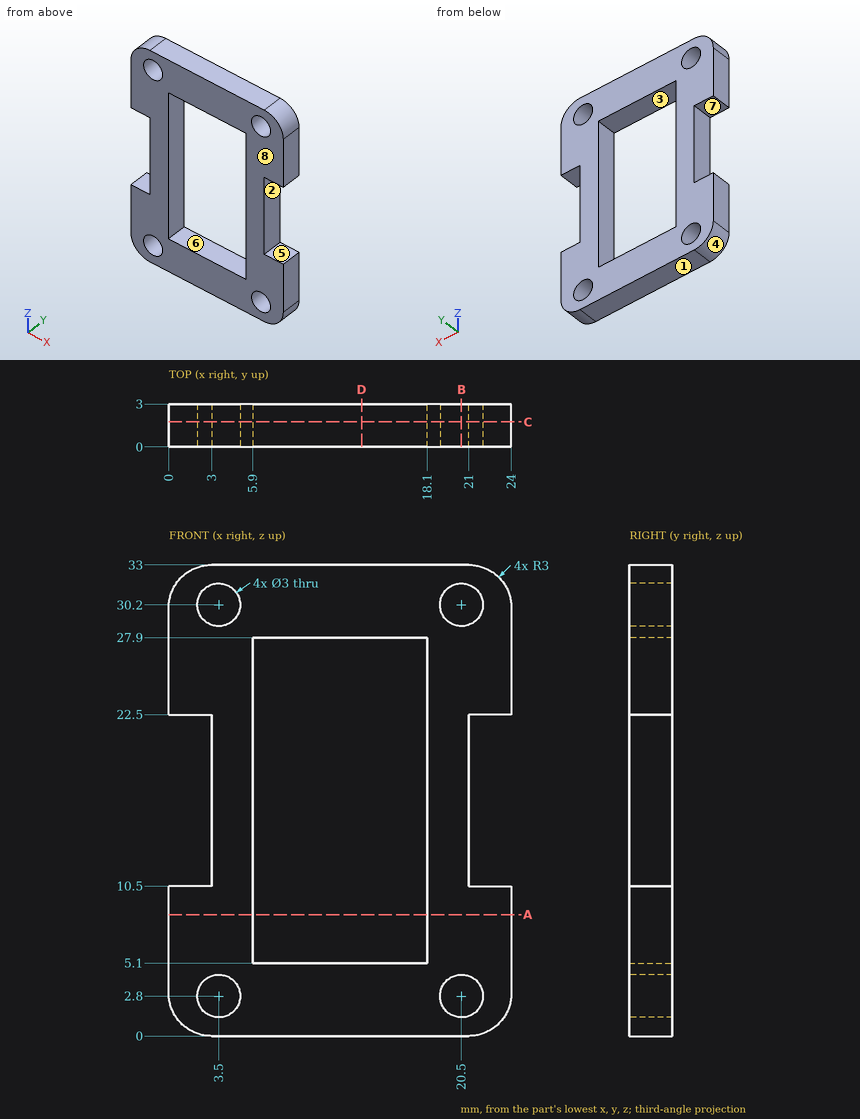
Could you check a few things on this drawing? It's one solid part, dimensions in mm from its lowest x, y, z. A direction names the side the tool comes from. Round coordinates to 2 decimals unless told otherwise and drop trailing zeros. Order: outer loops, then holes, each group sorted by start corner. A loop starts at its lowest first (then second) coordinate and runs counter-clockwise, first axis right, second up.
(1) Imagine slicing it at A-A (z = 8.5). Write out the boundary of the cut face in (x, y), plus the area to 3 significant figures.
Response values:
outline: (0, 0) - (5.9, 0) - (5.9, 3) - (0, 3) - close; (18.1, 0) - (24, 0) - (24, 3) - (18.1, 3) - close
area: 35.4 mm2
(2) Imagine slicing it at C-C (y = 1.75). Write out the boundary of the cut face in (x, z), plus the area to 3 significant figures.
Response values:
outline: (0, 3) arc R3 ccw to (3, 0) - (21, 0) arc R3 ccw to (24, 3) - (24, 10.5) - (21, 10.5) - (21, 22.5) - (24, 22.5) - (24, 30) arc R3 ccw to (21, 33) - (3, 33) arc R3 ccw to (0, 30) - (0, 22.5) - (3, 22.5) - (3, 10.5) - (0, 10.5) - close; hole circle Ø3 at (3.5, 2.8); hole circle Ø3 at (3.5, 30.2); hole (5.9, 5.1) - (18.1, 5.1) - (18.1, 27.9) - (5.9, 27.9) - close; hole circle Ø3 at (20.5, 2.8); hole circle Ø3 at (20.5, 30.2)
area: 406 mm2
(3) Imagine slicing it at D-D (x = 13.5). Write out the boundary of the cut face in (y, z).
Response values:
outline: (0, 0) - (3, 0) - (3, 5.1) - (0, 5.1) - close; (0, 27.9) - (3, 27.9) - (3, 33) - (0, 33) - close
(4) Imagine slicing it at B-B (x = 20.5). Write out the boundary of the cut face in (y, z).
Response values:
outline: (0, 0) - (3, 0) - (3, 1.3) - (0, 1.3) - close; (0, 4.3) - (3, 4.3) - (3, 28.7) - (0, 28.7) - close; (0, 31.7) - (3, 31.7) - (3, 33) - (0, 33) - close
(5) If we mould it in two halves opening along X, with no side actions, what happens to the marked faces 1, 2, 3 and 4? For each: released by +X, released by -X, zero draft, split by the parting line, or undercut.
Response values:
face 1: zero draft
face 2: released by +X
face 3: undercut
face 4: released by -X
(6) Please list where these lines run through material, in increasing order: line 1 along Z through (x, y) = (20.5, 2); line 2 along X through (y, z) = (0.65, 5.5); line 3 along X through (y, z) = (2, 15.5).
Response values:
line 1: z = 0 to 1.3, 4.3 to 28.7, 31.7 to 33
line 2: x = 0 to 5.9, 18.1 to 24
line 3: x = 3 to 5.9, 18.1 to 21
(7) Which directions (+Z, -Z, +X, -X, +Y, -Y) give clear straight access to the entire face, cutting with the end or side of a thin tool? Please do the marked faces 5, 6, 7 and 8.
Response values:
face 5: +X, +Y, -Y
face 6: +Y, -Y
face 7: -X, +Y, -Y
face 8: +Z, -Z, +X, -X, -Y
(8) I'm going to push flat-ended pins straight in: pin 1 (2 mm diameter, centred on x = 6, z = 9.5, fed in from -Y); pin 2 (1.5 mm diameter, centred on y = 1, z = 20.5, fed in from +X); pin 3 (0.9 mm diameter, centred on x = 23, y = 1, fed in from +Z); pin 4 (0.9 mm diameter, centred on y = 1, z = 17, fed in from -X). Where does each tip first touch, or does it pass through?
Response values:
pin 1: stops at y = 0
pin 2: stops at x = 21
pin 3: stops at z = 32.57
pin 4: stops at x = 3
